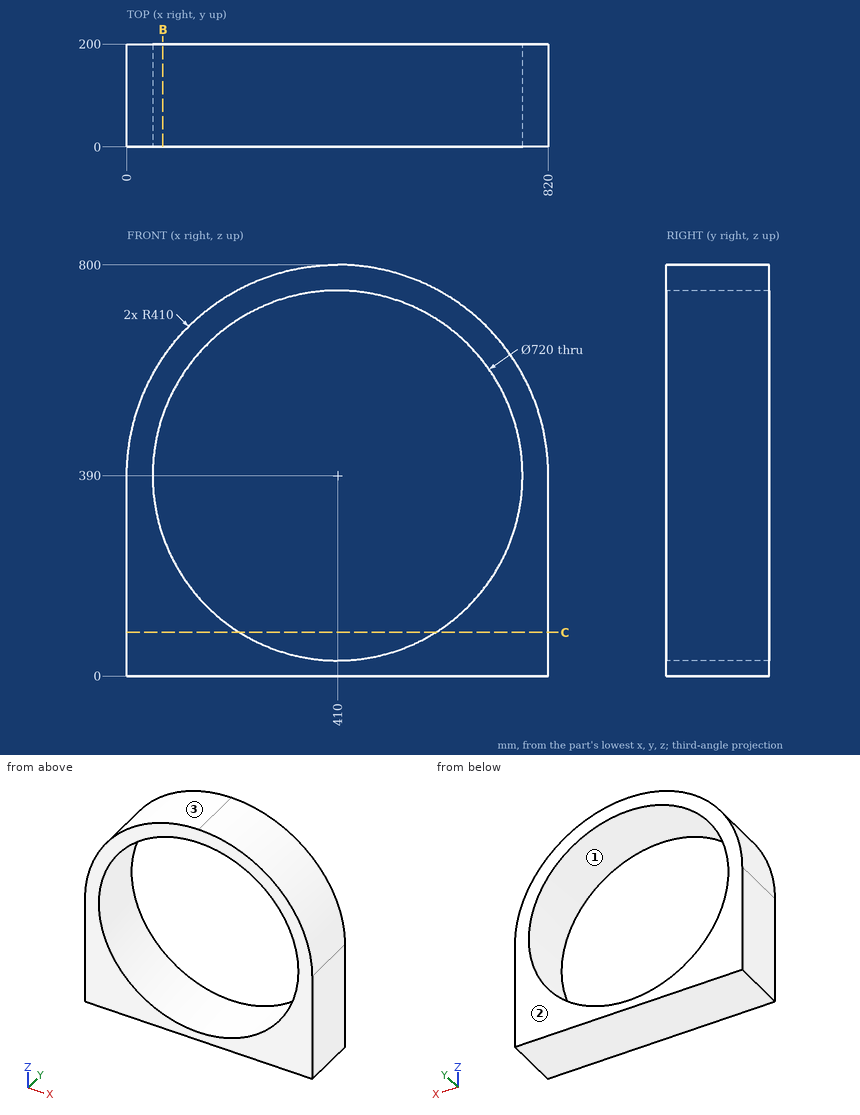
Print and shaded views of the part. All mm, measured from the part's lowest x, y and z. Coordinates: 2 decimals unless noted, no trailing zeros. Order: outer loops, then holes, each group sorted by start corner. A loop starts at its lowest first (then second) coordinate and runs counter-clockwise, first axis right, second up. Notation, with made-up numbers: (87, 75.5) -> (145, 75.5) arc R27 ccw to (145, 100.5) -> close; hole circle Ø11 at (83.5, 63.25). An arc over 180 degrees is marked (long way). Use one line per item in the form item = value. Start each with the question number.
1) Drop flat-ended pins along their axis: pin 1 (12 mm diameter, centred on x = 726, y = 99.5, fed in from +Z); pin 2 (10 mm diameter, centred on x = 693.5, y = 120, fed in from +Z) (1 decimal); pin 3 (10 mm diameter, centred on y = 145.5, z = 552.5, fed in from +X). Give the stop position or say it passes through.
2) Drill centre lines: L1, parallel to Z at x = 410, y = 155; L2, parallel to Z at x = 173, y = 168.5; L3, parallel to X at y = 92.5, z = 106.5 (1 decimal). Where is each one in solid material? Low to high. Write a range as [from, to].
3) Pull direction Z, two halves, no side cores. Call the marked faces 1, 2 and 3: +Z half, -Z half, draft (parallel to the pull), parting line (faces both ways), or undercut.
4) Band-saw the part on C-C on z = 85. Give the cut face in (x, y) (1 decimal).
5) Band-saw the part on B-B on x = 70. Give the cut face in (y, z).
Entries:
q1.pin_1 = 658.33
q1.pin_2 = 690.9
q1.pin_3 = 788.54
q2.L1 = [0, 30], [750, 800]
q2.L2 = [0, 119.02], [660.98, 724.56]
q2.L3 = [0, 188.1], [631.9, 820]
q3.face_1 = undercut
q3.face_2 = draft
q3.face_3 = +Z half
q4.outline = (0, 0) -> (218.8, 0) -> (218.8, 200) -> (0, 200) -> close; (601.2, 0) -> (820, 0) -> (820, 200) -> (601.2, 200) -> close
q5.outline = (0, 0) -> (200, 0) -> (200, 271.68) -> (0, 271.68) -> close; (0, 508.32) -> (200, 508.32) -> (200, 619.13) -> (0, 619.13) -> close
